The drawing under review shows one solid part. Ordinate dimensions are in mm from its lowest x, y, z. Round coordinates to 2 decimals unless told otherwise and drop trailing zeros. Write each loop counter-clockwise with the first axis right and the second up, starting at its lowest first coordinate (ties: lowest second). Pieces come first, ordered by that corner, then holes. Notation, with made-up numbers: (-21.5, 23.25) -> (18.5, 23.25) arc R12 ccw to (18.5, 35.25) -> close; hole circle Ø9 at (-3.75, 23.25). An arc over 180 degrees is marked (long way). Answer in a Markdown table with one row per item.
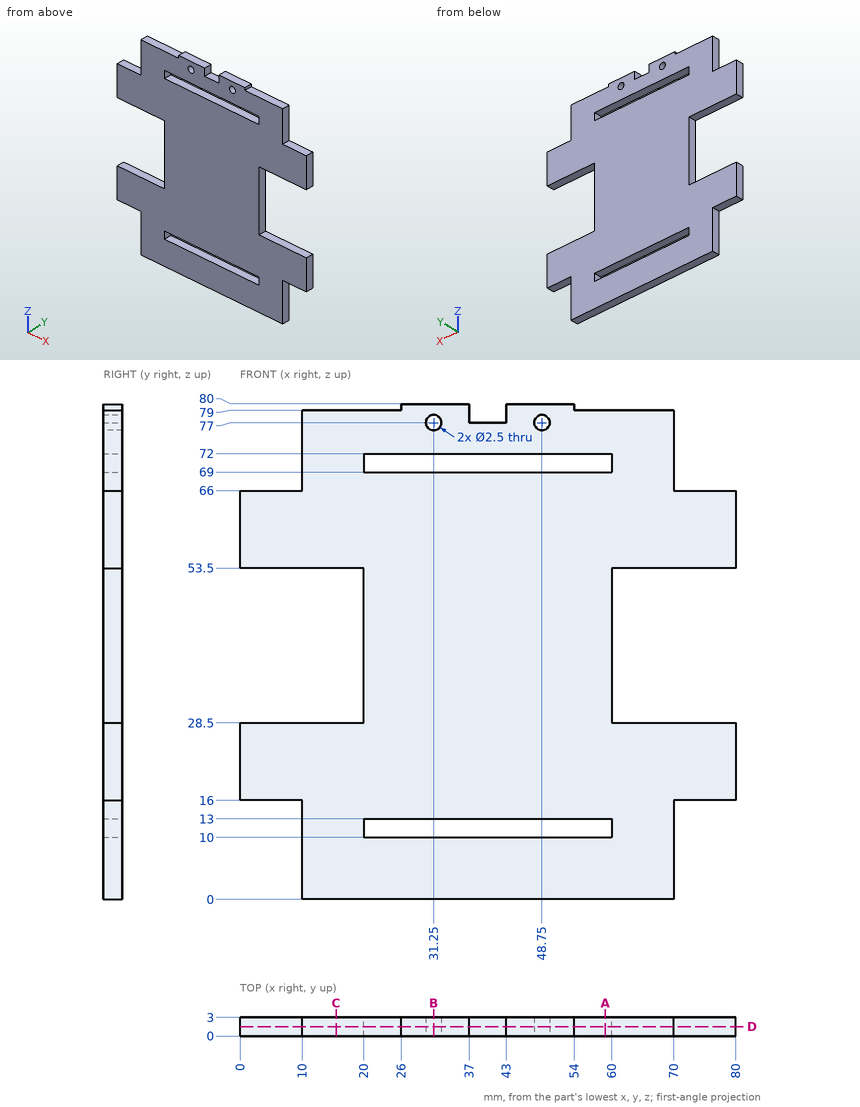
1) Consider section D-D on y = 1.5. State how many separate pieces and enclosed holes the cut face has, then the cut area to 3 significant figures.
Solved:
| item | result |
|---|---|
| separate pieces | 1 |
| enclosed holes | 4 |
| area | 4,500 mm² |
2) Consider section B-B on x = 31.25. State the section outline as (y, z) points.
Solved:
| item | result |
|---|---|
| outline | (0, 0) -> (3, 0) -> (3, 10) -> (0, 10) -> close; (0, 13) -> (3, 13) -> (3, 69) -> (0, 69) -> close; (0, 72) -> (3, 72) -> (3, 75.75) -> (0, 75.75) -> close; (0, 78.25) -> (3, 78.25) -> (3, 80) -> (0, 80) -> close |
3) Clearance check with flat-ended pins moving along their axes: pin 1 Ø0.9 at (y, z) = (1.5, 71) entering from +X; pin 2 Ø1.5 at (y, z) = (2, 53) entering from +X; pin 3 Ø0.9 at (y, z) = (1.5, 12) entering from -X; pin 4 Ø0.5 at (y, z) = (1, 79.5) entering from -X. State where each tip first meets the part, or that it passes through.
Solved:
| item | result |
|---|---|
| pin 1 | x = 70 |
| pin 2 | x = 80 |
| pin 3 | x = 10 |
| pin 4 | x = 26 |
4) Consider section C-C on x = 15.5. State the section outline as (y, z) points.
Solved:
| item | result |
|---|---|
| outline | (0, 0) -> (3, 0) -> (3, 28.5) -> (0, 28.5) -> close; (0, 53.5) -> (3, 53.5) -> (3, 79) -> (0, 79) -> close |
5) Consider section A-A on x = 59. State the section outline as (y, z) points, then the cut area to 3 significant figures.
Solved:
| item | result |
|---|---|
| outline | (0, 0) -> (3, 0) -> (3, 10) -> (0, 10) -> close; (0, 13) -> (3, 13) -> (3, 69) -> (0, 69) -> close; (0, 72) -> (3, 72) -> (3, 79) -> (0, 79) -> close |
| area | 219 mm² |
6) For line 1 (Z direction, x = 48.75, y = 1.8); line 2 (Z direction, x = 55, y = 2); line 3 (Z direction, x = 65, y = 1.8), list the stretches that pass through material, from the lowest coordinate up. Write a range as [from, to].
Solved:
| item | result |
|---|---|
| line 1 | [0, 10], [13, 69], [72, 75.75], [78.25, 80] |
| line 2 | [0, 10], [13, 69], [72, 79] |
| line 3 | [0, 28.5], [53.5, 79] |
